Here's how the part is built. I have some questions about the finished solid (model axes, mm). Face numbers are marked on the shaded views. A direction names the side the tool comes from. Coordinates: 2 decimals unless noted, no trailing zeros. Loops run counter-clockwise (first coordinate to the right, second up) from the corner with the lowest first, then second, coordinate; pieces in that order, holes last. Notation, with made-up numbers: (32.5, 16.25) -> (91.5, 16.25) arc R20 ccw to (91.5, 40.25) -> close; hole circle Ø7 at (39.25, 37.5). An arc over 180 degrees is marked (long way). Answer as a JSON object with one key per item and string values. Group by question number.
Q1. I want a section at D-D on y = -2.5. Write out the boundary of the cut face in (x, z), then the cut area to 3 significant figures.
Q2. I want a section at C-C on x = -27.94. Write out the boundary of the cut face in (y, z).
Q3. Thinking about a two-plate mould opening in Z: for the marked faces 5, 6 and 7, which applies, released by +Z, released by -Z, zero draft, split by the parting line, or undercut?
Q4. I want a section at B-B on y = -29.21. Write out the boundary of the cut face in (x, z), then the cut area to 3 significant figures.
Q5. I need wall thicknesses on line 1 (Y direction, x = -27.94, z = 3.05); line 2 (X direction, y = -29, z = 2); line 3 (Y direction, x = 10.5, z = 96). Which ranges of each line are inside material? Lowest first, please.
Q6. I'm going to push flat-ended pins straight in: pin 1 (4.5 mm diameter, centred on x = -18.5, z = 27, fed in from -Y); pin 2 (1.2 mm diameter, centred on x = -17.5, z = 26.5, fed in from +Y); pin 3 (2 mm diameter, centred on x = 1.5, z = 14, fed in from -Y); pin 4 (6 mm diameter, centred on x = -11, y = 22.5, fed in from -Z). Where does each tip first touch, or does it pass through?
Q7. I want a section at A-A on z = 14. Write out the boundary of the cut face in (x, y).
Q8. On a 3-axis mill with a long thin cutter (end or side, diameter ignored), from which of +Z, -Z, +X, -X, +Y, -Y can I reach the whole of each face in a straight line? I mean the marked faces 1, 2, 3 and 4. Say none if no direction works.
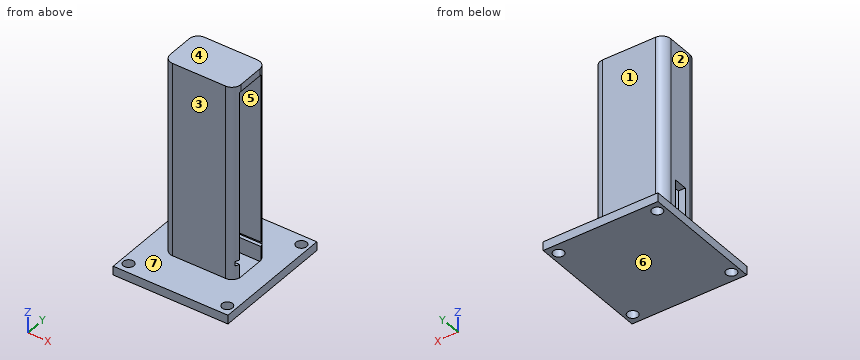
```python
from build123d import *

# Parameters (mm, degrees)
F0_W         = 65
F0_H         = 70
F1_DEPTH     = 5
F2_W         = 40
F2_H         = 25
F3_DEPTH     = 110
F5_D         = 6
F6_T         = -4
F7_W         = 7.9657556489
F7_H         = 25
F8_DEPTH     = 25
F10_DEPTH    = 2
F11_T1_DEPTH = 122.5


# Not quite as in the source:
# - a fillet or chamfer that OpenCascade refuses, or shapes differently, is made with other operations: its cross-section is extruded or revolved along the edge and cut away or added
# - a pattern or mirror of a feature is missing from the dataset's text; its kind, count and spacing are read off the source's solid


with BuildPart() as f1:
    # F0 (on Top) → F1 (new body)
    with BuildSketch(Plane.XY):
        Rectangle(F0_W, F0_H)
    extrude(amount=F1_DEPTH)

    # F2 (on face) → F3 (join)
    with BuildSketch(Plane.XY.offset(5)):
        Rectangle(F2_W, F2_H)
    extrude(amount=F3_DEPTH)

    # F5 (through all)
    with Locations(Plane(origin=(0, 0, 0), x_dir=(1, 0, 0), z_dir=(0, 0, -1))):
        with Locations((-27.94, 29.21), (27.94, 29.21), (27.94, -29.21), (-27.94, -29.21)):
            Hole(F5_D / 2)

    # F6: a shell. OpenCascade refuses it in one call, so the cavity is built on its own and cut out:
    # the body offset inwards by the wall thickness, plus a prism from it out through each open face.
    f6_core = offset(f1.part, amount=F6_T, kind=Kind.INTERSECTION, mode=Mode.PRIVATE)
    f6_exits = [f6_core.faces().sort_by_distance(p)[0] for p in [
        (16, 0, 57.5),
    ]]
    add(f6_core, mode=Mode.SUBTRACT)
    extrude(f6_exits, amount=-F6_T, mode=Mode.SUBTRACT)

    # F7 (on face) → F8 (cut)
    with BuildSketch(Plane.YZ.offset(-16)):
        with Locations((0, 24)):
            Rectangle(F7_W, F7_H)
    extrude(amount=-F8_DEPTH, mode=Mode.SUBTRACT)

    # F9 (on face) → F10 (cut)
    with BuildSketch(Plane.XZ.offset(-8.5)):
        with BuildLine():
            Line((20, 14), (20, 15.25))
            Line((20, 15.25), (-10, 15.25))
            ThreePointArc((-10, 15.25), (-11.25, 14), (-10, 12.75))
            Line((-10, 12.75), (20, 12.75))
            Line((20, 12.75), (20, 14))
        make_face()
    f10 = extrude(amount=-F10_DEPTH, mode=Mode.SUBTRACT)

    # F10_copies: F10 across plane
    add(f10.mirror(Plane(origin=(0, 0, 0), x_dir=(0, 0, -1), z_dir=(0, -1, 0))), mode=Mode.SUBTRACT)

    # F11: fillet of radius 5 on 4 edges, made by hand

    # F11_s2 → F11_t1 (cut)
    with BuildSketch(Plane.XY.offset(5)):
        with BuildLine():
            ThreePointArc((-15, -12.5), (-18.5355339059, -11.0355339059), (-20, -7.5))
            Line((-20, -7.5), (-20, -12.5))
            Line((-20, -12.5), (-15, -12.5))
        make_face()
        with BuildLine():
            ThreePointArc((-20, 7.5), (-18.5355339059, 11.0355339059), (-15, 12.5))
            Line((-15, 12.5), (-20, 12.5))
            Line((-20, 12.5), (-20, 7.5))
        make_face()
        with BuildLine():
            ThreePointArc((15, -12.5), (18.5355339059, -11.0355339059), (20, -7.5))
            Line((20, -7.5), (20, -12.5))
            Line((20, -12.5), (15, -12.5))
        make_face()
        with BuildLine():
            ThreePointArc((20, 7.5), (18.5355339059, 11.0355339059), (15, 12.5))
            Line((15, 12.5), (20, 12.5))
            Line((20, 12.5), (20, 7.5))
        make_face()
    extrude(amount=F11_T1_DEPTH, mode=Mode.SUBTRACT)


solid = f1.part
```
Result set:
{
 "1": {"outline": "(-32.5, 0) -> (32.5, 0) -> (32.5, 5) -> (20, 5) -> (20, 4) -> (-16, 4) -> (-16, 11.5) -> (-20, 11.5) -> (-20, 5) -> (-32.5, 5) -> close; (-20, 36.5) -> (-16, 36.5) -> (-16, 111) -> (20, 111) -> (20, 115) -> (-20, 115) -> close", "area": "773 mm²"},
 "2": {"outline": "(-35, 0) -> (-32.21, 0) -> (-32.21, 5) -> (-35, 5) -> close; (-26.21, 0) -> (26.21, 0) -> (26.21, 5) -> (-26.21, 5) -> close; (32.21, 0) -> (35, 0) -> (35, 5) -> (32.21, 5) -> close"},
 "3": {"face 5": "undercut", "face 6": "released by -Z", "face 7": "released by +Z"},
 "4": {"outline": "(-32.5, 0) -> (-30.94, 0) -> (-30.94, 5) -> (-32.5, 5) -> close; (-24.94, 0) -> (24.94, 0) -> (24.94, 5) -> (-24.94, 5) -> close; (30.94, 0) -> (32.5, 0) -> (32.5, 5) -> (30.94, 5) -> close", "area": "265 mm²"},
 "5": {"line 1": "y = -35 to -32.21, -26.21 to 26.21, 32.21 to 35", "line 2": "x = -32.5 to -30.93, -24.95 to 24.95, 30.93 to 32.5", "line 3": "y = -12.5 to -8.5, 8.5 to 12.5"},
 "6": {"pin 1": "stops at y = -12.34", "pin 2": "stops at y = 12.12", "pin 3": "stops at y = -12.5", "pin 4": "stops at z = 0"},
 "7": {"outline": "(-20, -7.5) arc R5 ccw to (-15, -12.5) -> (15, -12.5) arc R5 ccw to (19, -10.5) -> (-11.25, -10.5) -> (-11.25, -8.5) -> (-16, -8.5) -> (-16, -3.98) -> (-20, -3.98) -> close; (-20, 3.98) -> (-16, 3.98) -> (-16, 8.5) -> (-11.25, 8.5) -> (-11.25, 10.5) -> (19, 10.5) arc R5 ccw to (15, 12.5) -> (-15, 12.5) arc R5 ccw to (-20, 7.5) -> close"},
 "8": {"face 1": "+Z, +X, -X, +Y", "face 2": "+Z, -X, +Y, -Y", "face 3": "+Z, +X, -X, -Y", "face 4": "+Z, +X, -X, +Y, -Y"}
}
